from build123d import *

# Parameters (mm, degrees)
F0_W     = 17.78
F0_H     = 152.4
F1_DEPTH = 2.54
F3_DEPTH = 2.541
F5_DEPTH = 2.54


with BuildPart() as f1:
    # F0 (on Top) → F1 (new body)
    with BuildSketch(Plane.XY):
        with Locations((-8.043494, 67.378512)):
            Rectangle(F0_W, F0_H)
    extrude(amount=F1_DEPTH)

    # F2 (on face) → F3 (cut, through all)
    with BuildSketch(Plane.XY.offset(2.54)):
        with BuildLine():
            ThreePointArc((-8.043494, 139.768512), (-9.839545, 135.432461), (-5.503494, 137.228512))
            ThreePointArc((-5.503494, 137.228512), (-6.247443, 139.024564), (-8.043494, 139.768512))
        make_face()
    extrude(amount=-F3_DEPTH, mode=Mode.SUBTRACT)

    # F4 (on face) → F5 (join)
    with BuildSketch(Plane.XY.offset(2.54)):
        with BuildLine():
            ThreePointArc((-8.043494, -4.757488), (-6.427048, -4.087934), (-5.757494, -2.471488))
            ThreePointArc((-5.757494, -2.471488), (-9.65994, -0.855042), (-8.043494, -4.757488))
        make_face()
    extrude(amount=F5_DEPTH)


solid = f1.part
Geometry: final body of the model. Coordinates: model frame, mm. Round coordinates to 2 decimals unless told otherwise and drop trailing zeros. Order: outer loops, then holes, each group sorted by start corner. A loop starts at its lowest first (then second) coordinate and runs counter-clockwise, first axis right, second up.
Q1. Material intervals for probe 1 along Z at (x, y) = (-13.5, 103.5); probe 2 along Y at (x, z) = (-9.5, 1.85); probe 3 along Y at (x, z) = (-8.5, 0.95), sorted ascending.
Result sheet:
probe 1: z = 0 to 2.54
probe 2: y = -8.82 to 135.15, 139.31 to 143.58
probe 3: y = -8.82 to 134.73, 139.73 to 143.58
Q2. Section A-A, the plane y = 95.5. Output: boundary loops of the cut face in (x, z).
Result sheet:
outline: (-16.93, 0) - (0.85, 0) - (0.85, 2.54) - (-16.93, 2.54) - close
Q3. Section B-B, the plane x = -14. Output: boundary loops of the cut face in (y, z), and give its area (3 significant figures).
Result sheet:
outline: (-8.82, 0) - (143.58, 0) - (143.58, 2.54) - (-8.82, 2.54) - close
area: 387 mm2
Q4. Pin query (flat end, axial travel): pin 1 (6 mm diameter, centred on x = -14.5, y = 20.5, fed in from +Z). Return the tip coordinate at first contact, or that it passes through.
Result sheet:
pin 1: stops at z = 2.54
